```python
from build123d import *

# Parameters (mm, degrees)
F1_DEPTH = 38.1
F2_DEPTH = 25.4
F3_W     = 5.2324
F3_H     = 2.9972
F3_W_2   = 2.6162
F4_DEPTH = 12.7
F5_R     = 2.9972
F6_DEPTH = 38.1


with BuildPart() as f1:
    # F0 (on Front) → F1 (new body)
    with BuildSketch(Plane.XZ):
        Polygon((7.8359, 0), (-7.8359, 0), (-10.6045, -2.7686), (-9.2202, -4.1529), (-9.2075, -4.1656), (-7.8359, -5.5372), (-7.8359, -9.3218), (7.8359, -9.3218), (7.8359, -5.5372), (10.6045, -2.7686), align=None)
    extrude(amount=F1_DEPTH)

    # F0 (on Front) → F2 (join)
    with BuildSketch(Plane.XZ):
        Polygon((7.8359, 0), (-7.8359, 0), (-10.6045, -2.7686), (-9.2202, -4.1529), (-9.2075, -4.1656), (-7.8359, -5.5372), (-7.8359, -9.3218), (7.8359, -9.3218), (7.8359, -5.5372), (10.6045, -2.7686), align=None)
        Polygon((-9.2075, -4.1656), (-9.2202, -4.1529), (-9.2202, -4.1656), align=None)
    extrude(amount=F2_DEPTH)

    # F3 (on Right) → F4 (cut, symmetric)
    with BuildSketch(Plane.YZ):
        with Locations((-2.6162, -1.4986)):
            Rectangle(F3_W, F3_H)
        with Locations((-11.3157, -1.4986)):
            Rectangle(F3_W_2, F3_H)
        with Locations((-13.9319, -1.4986)):
            Rectangle(F3_W_2, F3_H)
        with Locations((-21.3233, -1.4986)):
            Rectangle(F3_W_2, F3_H)
        with Locations((-23.9395, -1.4986)):
            Rectangle(F3_W_2, F3_H)
        with Locations((-32.639, -1.4986)):
            Rectangle(F3_W, F3_H)
        with Locations((-42.6466, -1.4986)):
            Rectangle(F3_W, F3_H)
    extrude(amount=F4_DEPTH, both=True, mode=Mode.SUBTRACT)

    # F5 (on face) → F6 (cut)
    with BuildSketch(Plane(origin=(0, 0, 0), x_dir=(-1, 0, 0), z_dir=(0, 1, 0))):
        Circle(F5_R)
    extrude(amount=-F6_DEPTH, mode=Mode.SUBTRACT)


solid = f1.part
```
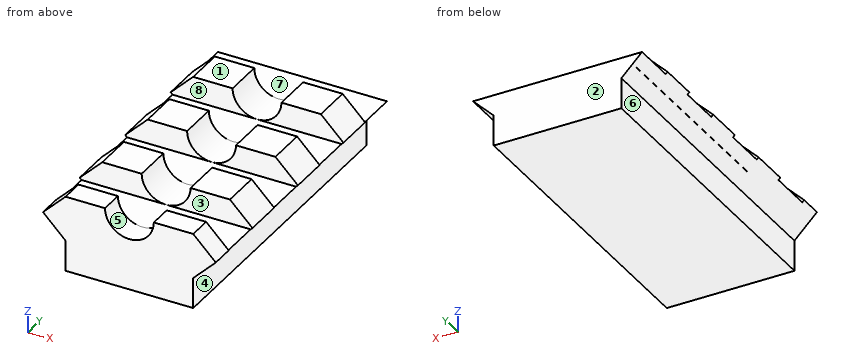
Source: CAD feature listing. Evaluate the final solid. Frame: model axes, mm. Face numbers are marked on the shaded views. A direction names the side the tool comes from. Round coordinates to 2 decimals unless told otherwise and drop trailing zeros. Loops run counter-clockwise (first coordinate to the right, second up) from the corner with the lowest first, then second, coordinate; pieces in that order, holes last. Notation, with made-up numbers: M 37,-7 L 86,-7 A27 ccw 86,32 Z; hole C 30,70.5 d6. An arc over 180 degrees is marked long. Use a Markdown table: item, result. Add a question column.
1. Cut plane B-B, the plane z = -1.25. State how many separate pieces and enclosed holes the cut face has, and give its area (3 significant figures).
2. Cut plane C-C, the plane x = -6.75. Output: boundary loops of the cut face in (y, z), and give its area (3 significant figures).
3. Contact query for flat-ended pins moving along their axis: pin 1 (1.5 mm diameter, centred on y = -25, z = -6.5, fed in from +X); pin 2 (4 mm diameter, centred on x = -2.5, y = -21.5, fed in from +Z); pin 3 (0.9 mm diameter, centred on x = -3, z = -1.5, fed in from +Y); pin 4 (1.6 mm diameter, centred on x = 0, y = -12, fed in from +Z). Output: stop coordinate, or through.
4. Ray query, line 1 along Y through (x, z) = (-4.5, -1.25); line 2 along X through (y, z) = (-18, -1.5); line 3 along Z through (x, y) = (7.5, -5). Return the intervals inside material, ascending. Write a range as [from, to].
5. Pull-direction query (Y, two-part tool) for the marked faces 1, 2 and 3; classes: +Y half, -Y half, draft (parallel to the pull), parting line (faces both ways), or undercut.
6. Cut plane A-A, the plane y = -27. Output: boundary loops of the cut face in (x, z).
7. Set-up query: the marked faces 4, 5, 6, 7 and 8. Return all of +Z, -Z, +X, -X, +Y, -Y with unobstructed straight access to the full face (end or side cutting, diameter ignored); none if empty.
Solution:
| question | item | result |
|---|---|---|
| 1 | separate pieces | 8 |
| 1 | enclosed holes | 0 |
| 1 | area | 218 mm2 |
| 2 | outline | M -38.1,-9.32 L 0,-9.32 L 0,-3 L -5.23,-3 L -5.23,0 L -10.01,0 L -10.01,-3 L -15.24,-3 L -15.24,0 L -20.02,0 L -20.02,-3 L -25.25,-3 L -25.25,0 L -30.02,0 L -30.02,-3 L -35.26,-3 L -35.26,0 L -38.1,0 Z |
| 2 | area | 292 mm2 |
| 3 | pin 1 | stops at x = 7.84 |
| 3 | pin 2 | stops at z = 0 |
| 3 | pin 3 | stops at y = -5.23 |
| 3 | pin 4 | stops at z = -3 |
| 4 | line 1 | y = [-38.1, -35.26], [-30.02, -25.25], [-20.02, -15.24], [-10.01, -5.23] |
| 4 | line 2 | x = [-9.34, -2.59], [2.59, 9.34] |
| 4 | line 3 | z = [-9.32, -3] |
| 5 | face 1 | draft |
| 5 | face 2 | +Y half |
| 5 | face 3 | undercut |
| 6 | outline | M -10.6,-2.77 L -7.84,-5.54 L -7.84,-9.32 L 7.84,-9.32 L 7.84,-5.54 L 10.6,-2.77 L 7.84,0 L 3,0 A3 cw -3,0 L -7.84,0 Z |
| 7 | face 4 | -Z, +X, +Y, -Y |
| 7 | face 5 | +Z, +Y, -Y |
| 7 | face 6 | -Z, -X, +Y, -Y |
| 7 | face 7 | +Z, +X, -X, +Y |
| 7 | face 8 | +Z, +X, -X |
